Read the model definition and answer for the solid it produces. Units are mm, in the model's axes. Face numbers are marked on the shaded views. A direction names the side the tool comes from. Give positions to 0.01 mm unless a question says otherwise; leave off trailing zeros. Order: outer loops, then holes, each group sorted by start corner. A loop starts at its lowest first (then second) coordinate and runs counter-clockwise, first axis right, second up. Notation, with made-up numbers: (-13, 29.25) - (12, 29.25) arc R23 ccw to (12, 47.25) - close; hole circle Ø3 at (88.25, 9). An arc over 180 degrees is marked (long way). Return JSON: item names as keys, results as strings.
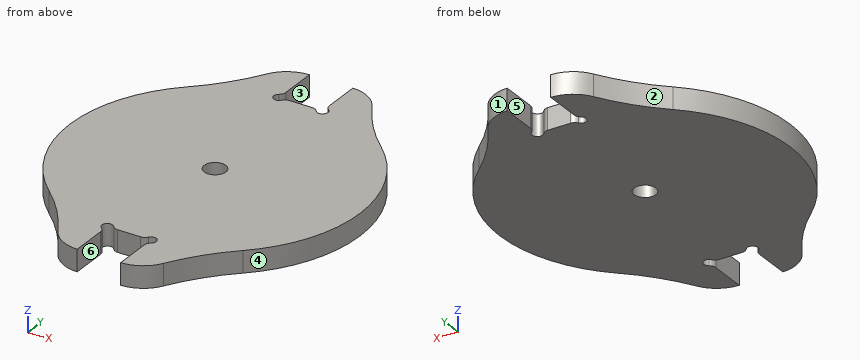
Autodesk Inventor part; units mm, degrees
ref_plane "YZ Plane" through (0, 0, 0) normal (1, 0, 0) x (0, 1, 0)
ref_plane "XZ Plane" through (0, 0, 0) normal (0, 1, 0) x (-1, 0, 0)
ref_plane "XY Plane" through (0, 0, 0) normal (0, 0, 1) x (1, 0, 0)
sketch "Sketch1" plane through (0, 0, 0) normal (0, 0, 1) x (1, 0, 0)
  circle A0 centre (0, 0) radius 1.5
  circle A1 centre (0, 0) radius 15.875 construction
  line L0 (0, 20) -> (0, -20) construction
  line L1 (-20, 0) -> (20, 0) construction
  line L2 (-2.25, 18.5) -> (0, 18.5)
  line L3 (-6, 25) -> (-3, 25)
  line L4 (-3, 25) -> (-3, 19.25)
  line L5 (2.25, 18.5) -> (0, 18.5)
  line L6 (6, 25) -> (3, 25)
  line L7 (3, 25) -> (3, 19.25)
  line L8 (-2.25, -18.5) -> (0, -18.5)
  line L9 (-6, -25) -> (-3, -25)
  line L10 (-3, -25) -> (-3, -19.25)
  line L11 (2.25, -18.5) -> (0, -18.5)
  line L12 (3, -25) -> (3, -19.25)
  line L13 (6, -25) -> (3, -25)
  arc A2 (-13.3625, 14.881) -> (-13.3625, -14.881) centre (0, 0) ccw
  arc A3 (13.3625, -14.881) -> (13.3625, 14.881) centre (0, 0) ccw
  circle A4 centre (0, 0) radius 20 construction
  arc A5 (-3, 19.25) -> (-2.25, 18.5) centre (-3, 18.5) ccw
  arc A6 (2.25, 18.5) -> (3, 19.25) centre (3, 18.5) ccw
  arc A7 (-2.25, -18.5) -> (-3, -19.25) centre (-3, -18.5) ccw
  arc A8 (3, -19.25) -> (2.25, -18.5) centre (3, -18.5) ccw
  arc A9 (-13.3625, 14.881) -> (-6, 25) centre (-33.4062, 37.2025) ccw
  arc A10 (6, 25) -> (13.3625, 14.881) centre (33.4062, 37.2025) ccw
  arc A11 (-6, -25) -> (-13.3625, -14.881) centre (-33.4062, -37.2025) ccw
  arc A12 (13.3625, -14.881) -> (6, -25) centre (33.4062, -37.2025) ccw
  dimension "d9" = 40
  dimension "d0" = 3
  dimension "d1" = 31.75
  dimension "GripLength" = 1.5
  dimension "d4" = 5
  dimension "d5" = 3
  dimension "d6" = 3
  dimension "d8" = 20
  dimension "d10" = 0.75
  dimension "d15" = 30
extrude "Extrusion1" add sketch "Sketch1" along normal blind 3
fillet "Fillet1" radius 1 8 edges at (-3, 19.25, 1.5) (-2.25, 18.5, 1.5) (2.25, 18.5, 1.5) (3, 19.25, 1.5) (-3, -19.25, 1.5) (-2.25, -18.5, 1.5) (2.25, -18.5, 1.5) (3, -19.25, 1.5)
fillet "Fillet2" radius 5 8 edges at (-13.3625, -14.881, 1.5) (-6, -25, 1.5) (6, -25, 1.5) (13.3625, -14.881, 1.5) (13.3625, 14.881, 1.5) (6, 25, 1.5) (-6, 25, 1.5) (-13.3625, 14.881, 1.5)
equation "\"d1\" = BattOD"
properties part number "Forward Endcap Outer"
Q1. A cutting plane is placed at D-D (x = -14.5). Write down the section's boundary in (y, z) (3 decimals).
Values:
{"outline": "(-13.775, 0) - (13.775, 0) - (13.775, 3) - (-13.775, 3) - close"}
Q2. A cutting plane is placed at A-A (x = 0). Write down the section's boundary in (y, z), and give its area (3 significant figures).
Values:
{"outline": "(-18.5, 0) - (-1.5, 0) - (-1.5, 3) - (-18.5, 3) - close; (1.5, 0) - (18.5, 0) - (18.5, 3) - (1.5, 3) - close", "area": "102 mm²"}
Q3. Determine the mould class of the marked faces 1, 2 and 3 for opening direction X: released by +X, released by -X, zero draft, split by the parting line, or undercut.
Values:
{"face 1": "released by +X", "face 2": "released by -X", "face 3": "undercut"}
Q4. Consider L1, parallel to X at y = -18, z = 0.2; L2, parallel to Y at x = 0.5, z = 2.3; L3, parallel to X at y = -22, z = 2.6. Determine where each line is inside the solid, lowest interval first.
Values:
{"L1": "x = -10.36 to -3.56, -2.44 to 2.44, 3.56 to 10.36", "L2": "y = -18.5 to -1.41, 1.41 to 18.5", "L3": "x = -7.54 to -3, 3 to 7.54"}
Q5. A cutting plane is placed at B-B (y = 0). Write down the section's boundary in (x, z).
Values:
{"outline": "(-20, 0) - (-1.5, 0) - (-1.5, 3) - (-20, 3) - close; (1.5, 0) - (20, 0) - (20, 3) - (1.5, 3) - close"}
Q6. For the marked faces 4, 5 and 6, determine the directions among +Z, -Z, +X, -X, +Y, -Y from which every point of the face is accessible in a straight line to the end or side of a thin tool.
Values:
{"face 4": "+Z, -Z, +X", "face 5": "+Z, -Z, +Y", "face 6": "+Z, -Z, -Y"}
Q7. Given pin 1 (1.5 mm diameter, centred on y = 23, z = 1.5, fed in from +X); pin 2 (1.5 mm diameter, centred on y = 22.5, z = 2, fed in from -X); pin 3 (1.5 mm diameter, centred on y = -23.5, z = 2, fed in from -X); pin 4 (1.2 mm diameter, centred on x = 3, y = -18.5, fed in from +Z), each flat-ended and moving along its own axis, determine where each tip first touches the part or whether it passes through.
Values:
{"pin 1": "stops at x = 7.4", "pin 2": "stops at x = -7.69", "pin 3": "stops at x = -7.1", "pin 4": "passes through"}
